For this review, use the dimensioned drawing (mm, ordinates from the lowest corner) and the shaded views. A direction names the side the tool comes from. Give positions to 0.01 mm unless a question says otherwise; leave off trailing zeros. Order: outer loops, then holes, each group sorted by start corner. A loop starts at its lowest first (then second) coordinate and runs counter-clockwise, first axis right, second up.
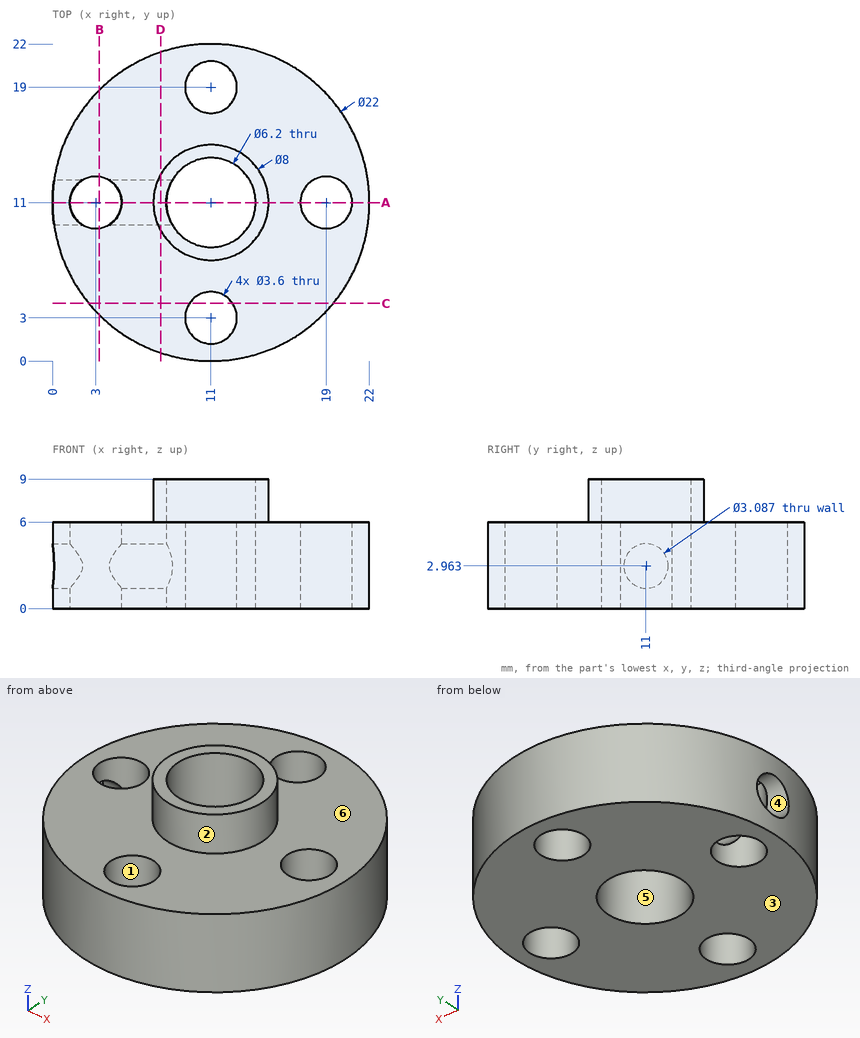
1. For line 1 along Y through (x, z) = (11, 2.8); line 2 along Z through (x, y) = (8.25, 2.5); line 3 along X through (y, z) = (20.5, 1.25) (1 decimal), list the stretches that pass through material, from the lowest coordinate up.
Recorded:
line 1: y = 0 to 1.2, 4.8 to 7.9, 14.1 to 17.2, 20.8 to 22
line 2: z = 0 to 6
line 3: x = 5.5 to 10, 12 to 16.5
2. Take a section at C-C (y = 4). State the section outline as (x, z) points (1 decimal).
Recorded:
outline: (2.5, 0) - (9.5, 0) - (9.5, 6) - (2.5, 6) - close; (12.5, 0) - (19.5, 0) - (19.5, 6) - (12.5, 6) - close
3. Machinability: for the marked faces 4, 5 and 6, which of the approach directions +Z, -Z, +X, -X, +Y, -Y give a long, thin tool a straight path to every point of the face, cutting with its end or side? Answer none if there is none.
Recorded:
face 4: -X
face 5: +Z, -Z
face 6: +Z
4. Draft analysis for pull direction Y (two halves, no side actions). For the marked faces 1, 2 and 3, state which applies: pulls with the +Y half, pulls with the -Y half, needs draft (parallel to the pull), parting line crosses it, or undercut.
Recorded:
face 1: undercut
face 2: parting line crosses it
face 3: needs draft
5. For pin 1 (3 mm diameter, centred on x = 19, y = 12, fed in from +Z); pin 2 (3 mm diameter, centred on y = 11, z = 2.96, fed in from -X); pin 3 (1.5 mm diameter, centred on x = 3, z = 5.5, fed in from -Y); pin 4 (2 mm diameter, centred on x = 11, y = 19, fed in from +Z), all flat-tipped, find the tip position at first contact; note any pin that passes through.
Recorded:
pin 1: stops at z = 6
pin 2: stops at x = 13.71
pin 3: stops at y = 2.73
pin 4: passes through
6. Take a section at A-A (y = 11). State the section outline as (x, z) points.
Recorded:
outline: (0, 0) - (1.2, 0) - (1.2, 1.42) - (0, 1.42) - close; (0, 4.51) - (1.2, 4.51) - (1.2, 6) - (0, 6) - close; (4.8, 0) - (7.9, 0) - (7.9, 1.42) - (4.8, 1.42) - close; (4.8, 4.51) - (7.9, 4.51) - (7.9, 9) - (7, 9) - (7, 6) - (4.8, 6) - close; (14.1, 0) - (17.2, 0) - (17.2, 6) - (15, 6) - (15, 9) - (14.1, 9) - close; (20.8, 0) - (22, 0) - (22, 6) - (20.8, 6) - close
7. Take a section at B-B (x = 3.25). State the section outline as (y, z) points.
Recorded:
outline: (3.19, 0) - (9.22, 0) - (9.22, 6) - (3.19, 6) - close; (12.78, 0) - (18.81, 0) - (18.81, 6) - (12.78, 6) - close
8. Take a section at D-D (x = 7.5). State the section outline as (y, z) points, then the cut area to 3 significant figures.
Recorded:
outline: (0.57, 0) - (21.43, 0) - (21.43, 6) - (12.94, 6) - (12.94, 9) - (9.06, 9) - (9.06, 6) - (0.57, 6) - close; hole circle Ø3.09 at (11, 2.96)
area: 129 mm2
